Here's the drawing with two shaded views (mm, measured from the low corner). I have some questions. A direction names the side the tool comes from. Coordinates: 2 decimals unless noted, no trailing zeros. Order: outer loops, then holes, each group sorted by start corner. A loop starts at its lowest first (then second) coordinate and runs counter-clockwise, first axis right, second up. Notation, with made-up numbers: (69.25, 37) -> (100.25, 37) arc R9 cw to (100.25, 48) -> close; hole circle Ø3 at (63.25, 39). An arc over 180 degrees is marked (long way). Write item = value, one per line.
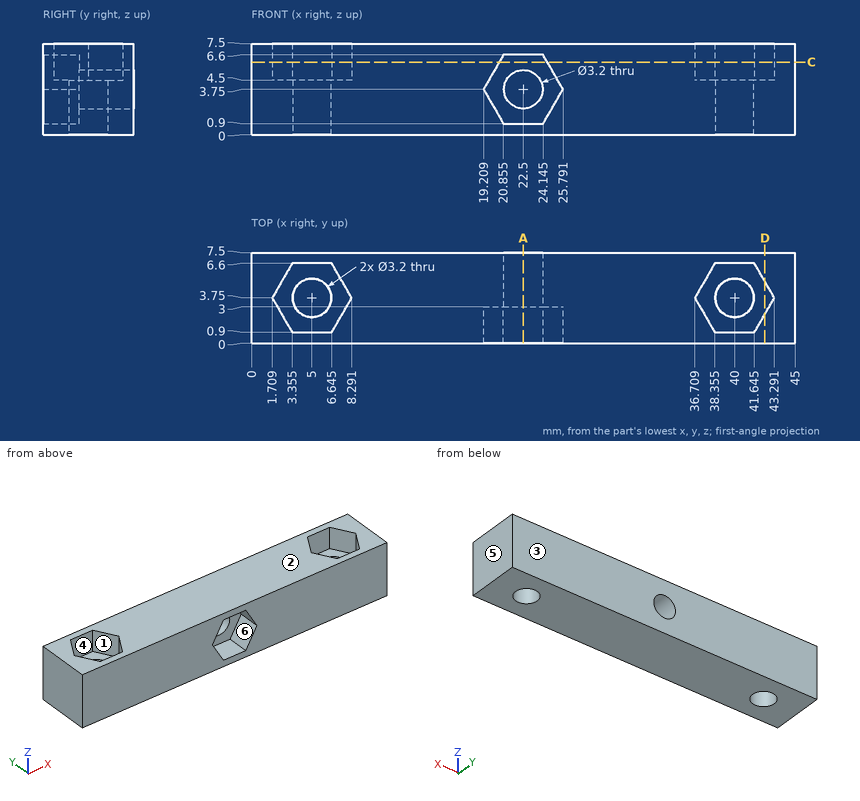
Item 1: If I drill on probe 1 along X at (y, z) = (3.75, 1.55); probe 2 along Y at (x, z) = (40, 1.3); probe 3 along X at (y, z) = (6, 6.75), over which ranges is the centre line in solid material (lowest first)?
A:
probe_1 = 0 to 3.4, 6.6 to 38.4, 41.6 to 45
probe_2 = 0 to 2.15, 5.35 to 7.5
probe_3 = 0 to 3.01, 6.99 to 38.01, 41.99 to 45
Item 2: If we mould it in two halves opening along Y, with no side actions, what happens to the marked faces 1, 2 and 3? For each: pulls with the +Y half, pulls with the -Y half, needs draft (parallel to the pull), parting line crosses it, or undercut.
A:
face_1 = undercut
face_2 = needs draft
face_3 = pulls with the +Y half
Item 3: For the marked faces 4, 5 and 6, which set-ups out of +Z, -Z, +X, -X, +Y, -Y let a thin tool reach every point of the face, with its end or its side?
A:
face_4 = +Z
face_5 = +Z, -Z, +X, +Y, -Y
face_6 = -Y
Item 4: I want a section at D-D, the plane x = 42.5. Please give me the cut outline in (y, z).
A:
outline = (0, 0) -> (7.5, 0) -> (7.5, 7.5) -> (5.12, 7.5) -> (5.12, 4.5) -> (2.38, 4.5) -> (2.38, 7.5) -> (0, 7.5) -> close
Item 5: I want a section at C-C, the plane z = 6. Give the number of separate pieces and of enclosed holes in the cut face, plus the area to 3 significant figures.
A:
separate_pieces = 1
enclosed_holes = 2
area = 269 mm2
Item 6: I want a section at A-A, the plane x = 22.5. Please give me the cut outline in (y, z).
A:
outline = (0, 0) -> (7.5, 0) -> (7.5, 2.15) -> (3, 2.15) -> (3, 0.9) -> (0, 0.9) -> close; (0, 6.6) -> (3, 6.6) -> (3, 5.35) -> (7.5, 5.35) -> (7.5, 7.5) -> (0, 7.5) -> close
